Part print with two shaded views. Sizes in mm from the minimum x, y, z corner. A direction names the side the tool comes from. Round coordinates to 2 decimals unless told otherwise and drop trailing zeros. Write each loop counter-clockwise with the first axis right and the second up, starting at its lowest first coordinate (ties: lowest second). Pieces come first, ordered by that corner, then holes. Notation, with made-up numbers: M -1,54.5 L 6,54.5 A26 ccw 6,82.5 Z; hole C 57.5,14 d10. An arc over 180 degrees is marked long. One line per question, with ' | ' between items. Start each with the question number.
1) Tool access for the marked faces 5 and 6: list every direction of +Z, -Z, +X, -X, +Y, -Y with a clear straight run to the whole face (end or side of a thin tool).
2) Drop flat-ended pins along their axis: pin 1 Ø5.5 at (x, z) = (25, 5) entering from -Y; pin 2 Ø3 at (x, y) = (9.5, 4) entering from +Z; pin 3 Ø3 at (x, y) = (10, 5) entering from +Z. Give the stop position or say it passes through.
3) Saw through at B-B (y = 5). List the corners of the cut face in (x, z), plus the area to 3 significant figures.
4) Mould opens along X. For the marked faces 1, 2, 3 and 4 say: pulls with the +X half, pulls with the -X half, needs draft (parallel to the pull), parting line crosses it, or undercut.
5) Saw through at D-D (z = 9). List the corners of the cut face in (x, y), plus the area to 3 significant figures.
6) Wall check: probe 1 along X at (y, z) = (5.25, 8.5); probe 2 along Y at (x, z) = (10, 7.2); probe 3 along X at (y, z) = (4, 1.25). Give the ranges that are in metal, low to high. Write a range as [from, to].
7) Saw through at A-A (z = 5). List the corners of the cut face in (x, y).
8) Saw through at C-C (x = 10). List the corners of the cut face in (y, z), plus the area to 3 significant figures.
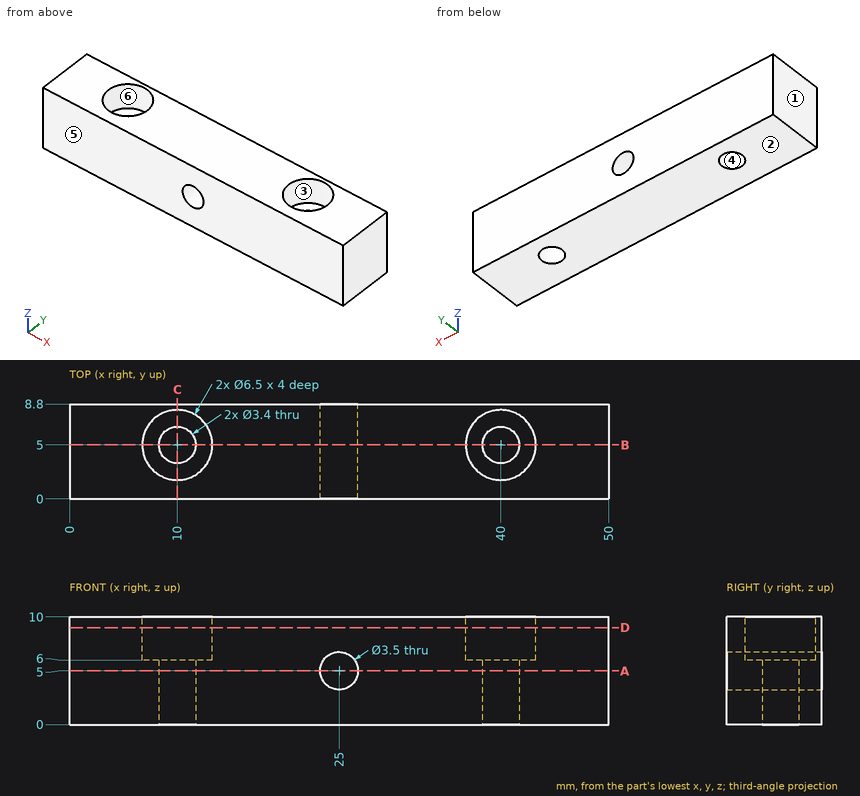
Answer key:
1) face 5: +Z, -Z, +X, -X, -Y | face 6: +Z
2) pin 1: stops at y = 0 | pin 2: stops at z = 6 | pin 3: passes through
3) outline: M 0,0 L 8.3,0 L 8.3,6 L 6.75,6 L 6.75,10 L 0,10 Z; M 11.7,0 L 38.3,0 L 38.3,6 L 36.75,6 L 36.75,10 L 13.25,10 L 13.25,6 L 11.7,6 Z; M 41.7,0 L 50,0 L 50,10 L 43.25,10 L 43.25,6 L 41.7,6 Z; hole C 25,5 d3.5 | area: 398 mm2
4) face 1: pulls with the -X half | face 2: needs draft | face 3: undercut | face 4: undercut
5) outline: M 0,0 L 50,0 L 50,8.8 L 0,8.8 Z; hole C 10,5 d6.5; hole C 40,5 d6.5 | area: 374 mm2
6) probe 1: x = [0, 6.76], [13.24, 36.76], [43.24, 50] | probe 2: y = [0, 1.75], [8.25, 8.8] | probe 3: x = [0, 8.63], [11.37, 38.63], [41.37, 50]
7) outline: M 0,0 L 23.25,0 L 23.25,8.8 L 0,8.8 Z; M 26.75,0 L 50,0 L 50,8.8 L 26.75,8.8 Z; hole C 10,5 d3.4; hole C 40,5 d3.4
8) outline: M 0,0 L 3.3,0 L 3.3,6 L 1.75,6 L 1.75,10 L 0,10 Z; M 6.7,0 L 8.8,0 L 8.8,10 L 8.25,10 L 8.25,6 L 6.7,6 Z | area: 41.6 mm2
